Can you work these out from the model? Positions are in its coordinate system, mm. Give positions to 0.01 mm unless a question says otherwise; leave off trailing zeros. Order: outer loops, then holes, each group sorted by start corner. A loop starts at its lowest first (then second) coordinate and runs counter-clockwise, first axis right, second up. Notation, with made-up numbers: (-28, 81) - (2, 81) arc R16 ccw to (2, 111) - close; hole circle Ø11 at (-27.75, -26.75). An arc over 180 degrees is marked (long way). Answer as a JSON object with one key per item and string values.
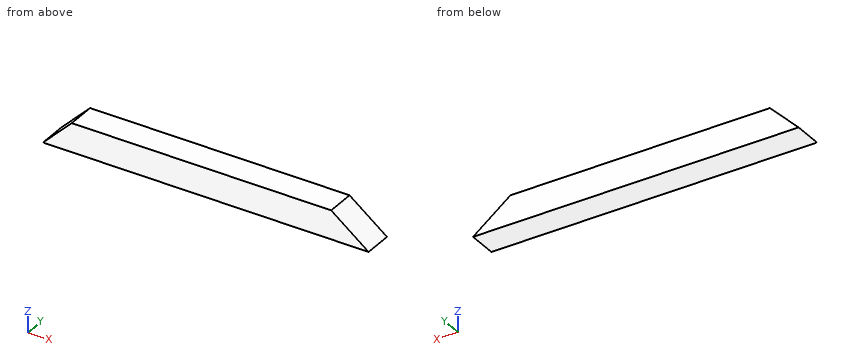
```python
from build123d import *

# Parameters (mm, degrees)
F1_DEPTH = 19.05
F2_SIZE  = 38.09999


# Not quite as in the source:
# - a fillet or chamfer is up to 0.001 mm smaller than in the source, because OpenCascade refuses the exact size


with BuildPart() as f1:
    # F0 (on Front) → F1 (new body, symmetric)
    with BuildSketch(Plane.XZ):
        Polygon((-215.9, 19.05), (-215.9, -19.05), (215.9, -19.05), (166.2471132948, 19.05), align=None)
    extrude(amount=F1_DEPTH, both=True)

    # F2 (size 38.1 in the source; OpenCascade refuses exactly that, so slightly less here)
    f2_edges = [f1.edges().sort_by_distance(p)[0] for p in [
        (-215.9, 0, 19.05),
    ]]
    chamfer(f2_edges, length=F2_SIZE)


solid = f1.part
```
Q1. I need wall thicknesses on L1, parallel to X at y = -5, z = -11; L2, parallel to X at y = -7, z = -13; L3, parallel to Z at x = 186, y = -8. Which ranges of each line are inside material? Lowest first, please.
Recorded:
{"L1": "x = -207.85 to 205.41", "L2": "x = -209.85 to 208.02", "L3": "z = -19.05 to 3.89"}
Q2. If we section it at C-C, the plane x = 182.5: Please give me the cut outline in (y, z).
Recorded:
{"outline": "(-19.05, -19.05) - (19.05, -19.05) - (19.05, 6.58) - (-19.05, 6.58) - close"}
Q3. I'm going to push flat-ended pins straight in: pin 1 Ø6 at (y, z) = (8.5, 3.5) entering from -X; pin 2 Ø1.5 at (y, z) = (-11, 11.5) entering from -X; pin 3 Ø10 at (y, z) = (2, 12.5) entering from -X. Where does each tip first touch, or does it pass through?
Recorded:
{"pin 1": "stops at x = -196.35", "pin 2": "stops at x = -186.1", "pin 3": "stops at x = -189.35"}
Q4. If we section it at B-B, the plane z = -11.5: Please give me the cut outline in (x, y).
Recorded:
{"outline": "(-208.35, -19.05) - (206.06, -19.05) - (206.06, 19.05) - (-208.35, 19.05) - close"}
